The drawing under review shows one solid part. Ordinate dimensions are in mm from its lowest x, y, z. A direction names the side the tool comes from. Round coordinates to 2 decimals unless told otherwise and drop trailing zeros. Order: outer loops, then holes, each group sorted by start corner. A loop starts at its lowest first (then second) coordinate and runs counter-clockwise, first axis right, second up. Notation, with made-up numbers: (24, 79) -> (56, 79) arc R24 cw to (56, 110) -> close; hole circle Ø3 at (55.5, 29.25). An arc over 180 degrees is marked (long way). Use a Markdown table: item, result. Add a question column.
1) Consider section A-A (x = 10). State the section outline as (y, z) points.
2) Clearance check with flat-ended pins moving along their axes: P1, Ø1, axis at x = 120.5, z = 2.5, coming from the +Y side; P2, Ø5.5, axis at y = 124.5, z = 7.5, coming from the -X side; P3, Ø8, axis at x = 20.5, z = 9.5, coming from the -Y side; P4, Ø1, axis at x = 82.5, z = 17, coming from the -Y side. State where each tip first meets the part, or that it passes through.
3) Consider section B-B (x = 67.5). State the section outline as (y, z) points, plus the area to 3 significant figures.
4) Wall thickness on line 1 along Y through (x, z) = (15.5, 16.75); line 2 along X through (y, z) = (224, 4.5): over which ranges is each line inside the solid? List them lowest first. Write a range as [from, to].
5) Draft analysis for pull direction Y (two halves, no side actions). For the marked faces 6, 7, 8 and 9, state which applies: pulls with the +Y half, pulls with the -Y half, needs draft (parallel to the pull), parting line crosses it, or undercut.
6) Machinability: for the marked faces 1, 2, 3, 4 and 5, which of the approach directions +Z, -Z, +X, -X, +Y, -Y give a long, thin tool a straight path to every point of the face, cutting with its end or side? Answer none if there is none.
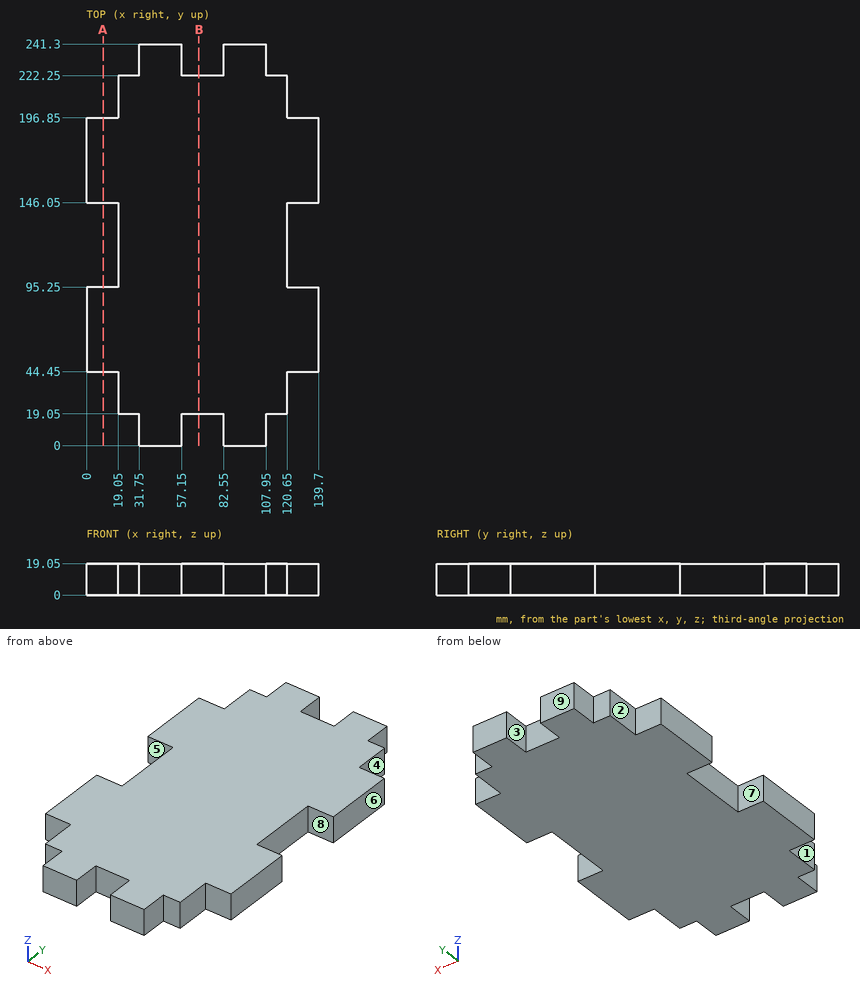
Results list:
| question | item | result |
|---|---|---|
| 1 | outline | (44.45, 0) -> (95.25, 0) -> (95.25, 19.05) -> (44.45, 19.05) -> close; (146.05, 0) -> (196.85, 0) -> (196.85, 19.05) -> (146.05, 19.05) -> close |
| 2 | P1 | y = 222.25 |
| 2 | P2 | x = 19.05 |
| 2 | P3 | y = 19.05 |
| 2 | P4 | y = 0 |
| 3 | outline | (19.05, 0) -> (222.25, 0) -> (222.25, 19.05) -> (19.05, 19.05) -> close |
| 3 | area | 3,870 mm2 |
| 4 | line 1 | [44.45, 95.25], [146.05, 196.85] |
| 4 | line 2 | [31.75, 57.15], [82.55, 107.95] |
| 5 | face 6 | needs draft |
| 5 | face 7 | undercut |
| 5 | face 8 | undercut |
| 5 | face 9 | pulls with the +Y half |
| 6 | face 1 | +Z, -Z, -X, -Y |
| 6 | face 2 | +Z, -Z, -X, +Y |
| 6 | face 3 | +Z, -Z, +Y |
| 6 | face 4 | +Z, -Z, +X, +Y |
| 6 | face 5 | +Z, -Z, -X |
